Part model, mm, in its own coordinate system. A direction names the side the tool comes from. Give positions to 0.01 mm unless a question says otherwise; leave off trailing zeros. Loops run counter-clockwise (first coordinate to the right, second up) from the corner with the lowest first, then second, coordinate; pieces in that order, holes last. Notation, with made-up numbers: (65.5, -31) -> (86.5, -31) arc R25 cw to (86.5, 7) -> close; hole circle Ø10 at (81, 67.25). An arc over 180 degrees is marked (long way). Write item = value, one per line.
Autodesk Fusion 360 part; units mm, degrees
sketch "Sketch1" plane through (0, 0, 0) normal (1, 0, 0) x (0, 1, 0)
  line L0 (0, 0) -> (40, 0)
  line L1 (40, 0) -> (40, 18)
  line L2 (40, 18) -> (0, 18)
  line L3 (0, 18) -> (0, 0)
  dimension "d1" = 40
  dimension "d2" = 18
extrude "Extrude1" add sketch "Sketch1" along normal blind 3
sketch "Sketch3" plane through (0, 0, 0) normal (0, 0, -1) x (1, 0, 0)
  line L0 (0, 0) -> (0, -40)
  line L1 (0, -40) -> (3, -40)
  line L2 (3, -40) -> (3, 0)
  line L3 (3, 0) -> (0, 0)
  line L4 (1.5, 0) -> (1.5, -40) construction
  line L5 (-15, -40) -> (10.4, -40)
  line L6 (10.4, -40) -> (10.4, 0)
  line L7 (10.4, 0) -> (-15, 0)
  line L8 (-15, 0) -> (-15, -40)
  dimension "d11" = 25.4
  dimension "d12" = 15
extrude "Extrude3" add sketch "Sketch3" along normal blind 3
fillet "Fillet1" radius 3 4 edges at (-15, 40, -1.5) (-15, 0, -1.5) (10.4, 0, -1.5) (10.4, 40, -1.5)
fillet "Fillet2" radius 1.5 2 edges at (1.5, 40, 18) (1.5, 0, 18)
fillet "Fillet3" radius 2 1 edges at (3, 20, 0)
fillet "Fillet4" radius 0.5 1 edges at (0, 20, 0)
1) Slice it at A-A, the plane y = 23. List the corners of the cut face in (x, z), and give its area (3 significant figures).
Resolved:
outline = (-15, -3) -> (10.4, -3) -> (10.4, 0) -> (5, 0) arc R2 cw to (3, 2) -> (3, 18) -> (0, 18) -> (0, 0.5) arc R0.5 cw to (-0.5, 0) -> (-15, 0) -> close
area = 131 mm²
2) Drop flat-ended pins along their axis: P1, Ø5, axis at y = 7, z = 5, coming from the +X side; P2, Ø5, axis at y = 9.5, z = 12.5, coming from the -X side; P3, Ø11.5, axis at x = -6.5, y = 11, coming from the +Z side. Give the stop position or say it passes through.
Resolved:
P1 = 3
P2 = 0
P3 = 0
3) Drill centre lines: line 1 along Z through (x, y) = (-3.25, 31); line 2 along X through (y, z) = (23.5, 2); line 3 along Y through (x, z) = (2, 16.75). Where is each one in solid material? Low to high. Write a range as [from, to].
Resolved:
line_1 = [-3, 0]
line_2 = [0, 3]
line_3 = [0.02, 39.98]
4) Which spindle directions (+Z, -Z, +X, -X, +Y, -Y) get a long thin tool onto all of the face, cutting with end or side? Do faces 1 (the face through (8, 20, 0)), 2 (the face through (-8, 20, 0)), 3 (the face through (9.54, 0.9, -1.52)). Say none if no direction does.
Resolved:
face_1 = +Z, +X, +Y, -Y
face_2 = +Z, -X, +Y, -Y
face_3 = +Z, -Z, +X, -Y
5) Slice it at B-B, the plane z = 4.25. List the corners of the cut face in (x, y), and give its area (3 significant figures).
Resolved:
outline = (0, 0) -> (3, 0) -> (3, 40) -> (0, 40) -> close
area = 120 mm²
6) Slice it at C-C, the plane x = -7.25. List the corners of the cut face in (y, z).
Resolved:
outline = (0, -3) -> (40, -3) -> (40, 0) -> (0, 0) -> close
